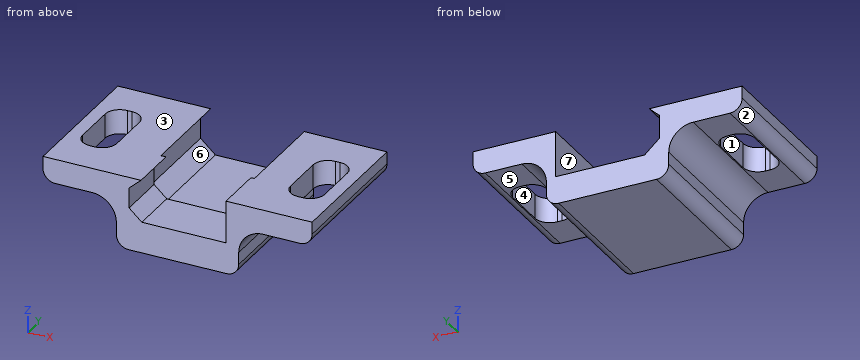
Solid Edge part; units mm, degrees
sketch "Sketch1" plane through (0, 0, 0) normal (0, -1, 0) x (1, 0, 0)
  line L0 (12.5, -7.5) -> (12.5, -2.5)
  arc A0 (17.5, 2.5) -> (12.5, -2.5) centre (17.5, -2.5) ccw
  line L1 (17.5, 2.5) -> (27.5, 2.5)
  line L2 (27.5, 2.5) -> (27.5, 7.5)
  line L3 (27.5, 7.5) -> (12.5, 7.5)
  line L4 (12.5, 7.5) -> (-12.5, 7.5)
  line L5 (-12.5, 7.5) -> (-27.5, 7.5)
  line L6 (-27.5, 7.5) -> (-27.5, 2.5)
  line L7 (-27.5, 2.5) -> (-17.5, 2.5)
  arc A1 (-17.5, 2.5) -> (-12.5, -2.5) centre (-17.5, -2.5) cw
  line L8 (-12.5, -2.5) -> (-12.5, -7.5)
  line L9 (-12.5, -7.5) -> (12.5, -7.5)
extrude "Protrusion1" add sketch "Sketch1" against normal blind 30
sketch "Sketch2" plane through (0, 0, 0) normal (0, -1, 0) x (1, 0, 0)
  line L0 (-9.9, 5.3168) -> (-7.4742, 7.5)
  line L1 (-7.25, 7.5) -> (-7.4742, 7.5)
  line L2 (-7.25, 7.5) -> (0, 7.5)
  line L3 (0, 7.5) -> (9.75, 7.5)
  line L4 (-7.4742, 7.5) -> (9.9, 7.5)
  line L5 (9.9, 7.5) -> (9.9, -1.15)
  line L6 (9.9, -1.15) -> (-7.3076, -1.15)
  line L7 (-7.3076, -1.15) -> (-9.9, 1.1832)
  line L8 (-9.9, 1.1832) -> (-9.9, 5.3168)
extrude "Cutout1" cut sketch "Sketch2" against normal blind 11 material side at (-8.6537, 0, 6.3712)
sketch "Sketch3" plane through (0, 30, 0) normal (0, 1, 0) x (-1, 0, 0)
  line L0 (-10.6, 7.5) -> (8.5206, 7.5)
  line L1 (10.6, 5.6286) -> (8.5206, 7.5)
  line L2 (10.6, 0.8714) -> (10.6, 5.6286)
  line L3 (7.5762, -1.85) -> (10.6, 0.8714)
  line L4 (-10.6, -1.85) -> (7.5762, -1.85)
  line L5 (-10.6, 7.5) -> (-10.6, -1.85)
extrude "Cutout2" cut sketch "Sketch3" against normal blind 20
fillet "Round1" radius 2.5 4 edges at (-27.5, 15, 2.5) (27.5, 15, 2.5) (12.5, 15, -7.5) (-12.5, 15, -7.5)
sketch "Sketch4" plane through (-21.25, 15, 2.5) normal (0, 0, -1) x (1, 0, 0)
  line L0 (-3.5, 4.5) -> (-3.5, -4.5)
  arc A0 (-3.5, -4.5) -> (-0.5, -7.5) centre (-0.5, -4.5) ccw
  line L1 (-0.5, -7.5) -> (0.5, -7.5)
  arc A1 (0.5, -7.5) -> (3.5, -4.5) centre (0.5, -4.5) ccw
  line L2 (3.5, -4.5) -> (3.5, 4.5)
  arc A2 (0.5, 7.5) -> (3.5, 4.5) centre (0.5, 4.5) cw
  line L3 (0.5, 7.5) -> (-0.5, 7.5)
  arc A3 (-0.5, 7.5) -> (-3.5, 4.5) centre (-0.5, 4.5) ccw
  line L4 (39, 4.5) -> (39, -4.5)
  arc A4 (42, -7.5) -> (39, -4.5) centre (42, -4.5) cw
  line L5 (42, -7.5) -> (43, -7.5)
  arc A5 (43, -7.5) -> (46, -4.5) centre (43, -4.5) ccw
  line L6 (46, -4.5) -> (46, 4.5)
  arc A6 (46, 4.5) -> (43, 7.5) centre (43, 4.5) ccw
  line L7 (43, 7.5) -> (42, 7.5)
  arc A7 (42, 7.5) -> (39, 4.5) centre (42, 4.5) ccw
extrude "Cutout3" cut sketch "Sketch4" against normal blind 10
Verification items for the finished model (mm, model axes). Face numbers are marked on the shaded views. A direction names the side the tool comes from. Coordinates: 2 decimals unless noted, no trailing zeros. Loops run counter-clockwise (first coordinate to the right, second up) from the corner with the lowest first, then second, coordinate; pieces in that order, holes last. Notation, with made-up numbers: (83.25, 24) - (135.25, 24) arc R5 ccw to (135.25, 28) - close; hole circle Ø3 at (-40, 25). An arc over 180 degrees is marked (long way). Answer as a JSON object with one key per item and string values.
(1) Access from +Z, -Z, +X, -X, +Y, -Y to the whole of each face (thin tool, end or side, straight path). Record for the marked faces 4, 5, 6 and 7.
Response:
{"face 4": "+Z, -Z", "face 5": "-Z, +X, +Y, -Y", "face 6": "+Y", "face 7": "+Z, +Y"}
(2) Cross-section at A-A, the plane z = 3.5. Record the boundary of the cut face in (x, y), then the cut area to 3 significant figures.
Response:
{"outline": "(-27, 0) - (-9.9, 0) - (-9.9, 10) - (-10.6, 10) - (-10.6, 30) - (-27, 30) - close; (9.9, 0) - (27, 0) - (27, 30) - (10.6, 30) - (10.6, 10) - (9.9, 10) - close; hole (-24.75, 10.5) arc R3 ccw to (-21.75, 7.5) - (-20.75, 7.5) arc R3 ccw to (-17.75, 10.5) - (-17.75, 19.5) arc R3 ccw to (-20.75, 22.5) - (-21.75, 22.5) arc R3 ccw to (-24.75, 19.5) - close; hole (17.75, 10.5) arc R3 ccw to (20.75, 7.5) - (21.75, 7.5) arc R3 ccw to (24.75, 10.5) - (24.75, 19.5) arc R3 ccw to (21.75, 22.5) - (20.75, 22.5) arc R3 ccw to (17.75, 19.5) - close", "area": "803 mm²"}
(3) Cross-section at C-C, the plane x = 19.5. Record the boundary of the cut face in (y, z).
Response:
{"outline": "(0, 2.5) - (7.77, 2.5) - (7.77, 7.5) - (0, 7.5) - close; (22.23, 2.5) - (30, 2.5) - (30, 7.5) - (22.23, 7.5) - close"}
(4) Mould release check, pull along X, two halves, no side actions. Record for the marked faces 1, 2 and 3: pulls with the +X half, pulls with the -X half, needs draft (parallel to the pull), parting line crosses it, or undercut.
Response:
{"face 1": "undercut", "face 2": "pulls with the -X half", "face 3": "needs draft"}
(5) Go/stop test with flat-tipped pins: pin 1 Ø2 at (y, z) = (15.5, -3.5) entering from +X; pin 2 Ø2 at (x, y) = (14.5, 22.5) entering from -Z; pin 3 Ø3 at (x, y) = (2.5, 3.5) entering from +Z. Record where each tip stops, or that it passes through.
Response:
{"pin 1": "stops at x = 12.5", "pin 2": "stops at z = 0.5", "pin 3": "stops at z = -1.15"}
(6) Scan lines: line 1 along Z through (x, y) = (7.5, 21); line 2 along X through (y, z) = (9.5, 3.25); line 3 along X through (y, z) = (14.25, -1). Record each from-to range of solid material in increasing order.
Response:
{"line 1": "z = -7.5 to -1.85", "line 2": "x = -26.79 to -24.58, -17.92 to -9.9, 9.9 to 17.92, 24.58 to 26.79", "line 3": "x = -12.73 to -8.52, 10.6 to 12.73"}
(7) Cross-section at D-D, the plane y = 5. Record the boundary of the cut face in (x, z).
Response:
{"outline": "(-27.5, 5) arc R2.5 ccw to (-25, 2.5) - (-17.5, 2.5) arc R5 cw to (-12.5, -2.5) - (-12.5, -5) arc R2.5 ccw to (-10, -7.5) - (10, -7.5) arc R2.5 ccw to (12.5, -5) - (12.5, -2.5) arc R5 cw to (17.5, 2.5) - (25, 2.5) arc R2.5 ccw to (27.5, 5) - (27.5, 7.5) - (9.9, 7.5) - (9.9, -1.15) - (-7.31, -1.15) - (-9.9, 1.18) - (-9.9, 5.32) - (-7.47, 7.5) - (-27.5, 7.5) - close"}
(8) Cross-section at B-B, the plane y = 17.5. Record the boundary of the cut face in (x, z), then the cut area to 3 significant figures.
Response:
{"outline": "(-27.5, 5) arc R2.5 ccw to (-25, 2.5) - (-24.75, 2.5) - (-24.75, 7.5) - (-27.5, 7.5) - close; (-17.75, 2.5) - (-17.5, 2.5) arc R5 cw to (-12.5, -2.5) - (-12.5, -5) arc R2.5 ccw to (-10, -7.5) - (10, -7.5) arc R2.5 ccw to (12.5, -5) - (12.5, -2.5) arc R5 cw to (17.5, 2.5) - (17.75, 2.5) - (17.75, 7.5) - (10.6, 7.5) - (10.6, -1.85) - (-7.58, -1.85) - (-10.6, 0.87) - (-10.6, 5.63) - (-8.52, 7.5) - (-17.75, 7.5) - close; (24.75, 2.5) - (25, 2.5) arc R2.5 ccw to (27.5, 5) - (27.5, 7.5) - (24.75, 7.5) - close", "area": "268 mm²"}
